Check sheet for the modelled part. Datum: model origin and axes. Units: mm. Face numbers are marked on the shaded views. A direction names the side the tool comes from. Round coordinates to 2 decimals unless told otherwise and drop trailing zeros. Order: outer loops, then holes, each group sorted by start corner. A loop starts at its lowest first (then second) coordinate and runs counter-clockwise, first axis right, second up.
Q1. Set-up check for the marked faces 1 and 2: record each of +Z, -Z, +X, -X, +Y, -Y from which the full face is reachable in a straight line by a thin tool's end or side.
Q2. Scan lines: probe 1 along Y at (x, z) = (12.7, -2.6); probe 2 along Y at (x, z) = (12, -1); probe 3 along Z at (x, y) = (41, -46). Record each from-to range of solid material in increasing order.
Q3. Cross-section at B-B on x = 139.7. Record the cut outline in (y, z).
Q4. Depth check by flat-ended pin: P1, Ø8, axis at x = 88.9, y = -19.23, coming from the -Z side; P2, Ø10, axis at x = 52.5, y = -10, coming from the -Z side; P3, Ø5, axis at x = 21.5, z = -19.5, coming from the -Y side; P4, Ø3, axis at x = 12.7, y = -19.23, coming from the -Z side. Enter the tip coordinate at first touch or a pass-through.
Q5. Cross-section at D-D on x = 41.5. Record the cut outline in (y, z).
Q6. Cross-section at C-C on y = -33. Record the cut outline in (x, z), then the cut area to 3 significant figures.
Q7. Cross-section at A-A on x = 12.7. Record the cut outline in (y, z).
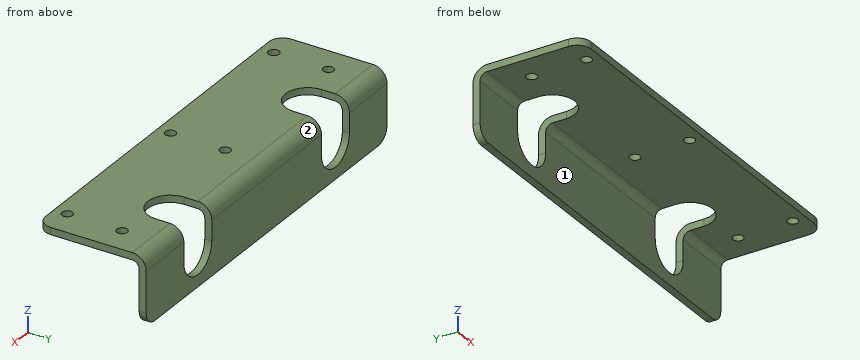
from build123d import *

# Parameters (mm, degrees)
BASE_FLANGE1_DEPTH           = 177.8
CUT_EXTRUDE1_DEPTH           = 6.5278
F_10_0_1935_DIAMETER_HOLE1_D = 4.9149
FILLET1_R                    = 6.35
CUT_EXTRUDE2_DEPTH           = 3.2639


# Sheet-metal steps are written as plain solids
with BuildPart() as part:
    # Sketch1 → Base-Flange1 (new body)
    with BuildSketch(Plane(origin=(0, 0, 0), x_dir=(0, 0, -1), z_dir=(1, 0, 0))):
        with BuildLine():
            Line((31.75, 0), (6.5278, 0))
            ThreePointArc((6.5278, 0), (1.911948354, -1.911948354), (0, -6.5278))
            Line((0, -6.5278), (0, -50.8))
            Line((0, -50.8), (3.2639, -50.8))
            Line((3.2639, -50.8), (3.2639, -6.5278))
            ThreePointArc((3.2639, -6.5278), (4.219874177, -4.219874177), (6.5278, -3.2639))
            Line((6.5278, -3.2639), (31.75, -3.2639))
            Line((31.75, -3.2639), (31.75, 0))
        make_face()
    extrude(amount=BASE_FLANGE1_DEPTH)

    # Sketch6 → Cut-Extrude1 (cut)
    with BuildSketch(Plane(origin=(0, 0, 0), x_dir=(1, 0, 0), z_dir=(0, 1, 0))):
        with BuildLine():
            Line((27.78125, 0), (27.78125, 15.875))
            ThreePointArc((27.78125, 15.875), (38.1, 26.19375), (48.41875, 15.875))
            Line((48.41875, 15.875), (48.41875, 0))
            ThreePointArc((48.41875, 0), (38.1, -10.31875), (27.78125, 0))
        make_face()
        with BuildLine():
            Line((129.38125, 0), (129.38125, 15.875))
            ThreePointArc((129.38125, 15.875), (139.7, 26.19375), (150.01875, 15.875))
            Line((150.01875, 15.875), (150.01875, 0))
            ThreePointArc((150.01875, 0), (139.7, -10.31875), (129.38125, 0))
        make_face()
    extrude(amount=-CUT_EXTRUDE1_DEPTH, mode=Mode.SUBTRACT)

    # #10 (0.1935) Diameter Hole1 (through all)
    with Locations(Plane.XY):
        with Locations((12.7, -19.2278), (88.9, -19.2278), (165.1, -19.2278), (88.9, -44.6278), (165.1, -44.6278), (12.7, -44.6278)):
            Hole(F_10_0_1935_DIAMETER_HOLE1_D / 2)

    # Fillet1
    fillet1_edges = [part.edges().sort_by_distance(p)[0] for p in [
        (177.8, -50.8, -1.63195),
        (0, -50.8, -1.63195),
        (177.8, -1.63195, -31.75),
        (0, -1.63195, -31.75),
    ]]
    fillet(fillet1_edges, radius=FILLET1_R)

    # Sketch9 → Cut-Extrude2 (cut)
    with BuildSketch(Plane.XY):
        with BuildLine():
            Line((48.41875, -6.5278), (48.41875, -12.8778))
            ThreePointArc((48.41875, -12.8778), (38.1, -23.19655), (27.78125, -12.8778))
            Line((27.78125, -12.8778), (27.78125, -6.5278))
            ThreePointArc((27.78125, -6.5278), (38.1, 3.79095), (48.41875, -6.5278))
        make_face()
        with BuildLine():
            Line((150.01875, -6.5278), (150.01875, -12.8778))
            ThreePointArc((150.01875, -12.8778), (139.7, -23.19655), (129.38125, -12.8778))
            Line((129.38125, -12.8778), (129.38125, -6.5278))
            ThreePointArc((129.38125, -6.5278), (139.7, 3.79095), (150.01875, -6.5278))
        make_face()
    extrude(amount=-CUT_EXTRUDE2_DEPTH, mode=Mode.SUBTRACT)


solid = part.part
Results found:
1. face 1: -Z, +X, -X, -Y
1. face 2: +Z, +X, -X, +Y
2. probe 1: y = -50.8 to -47.09, -42.17 to -21.69, -16.77 to -1.31
2. probe 2: y = -50.8 to -46.98, -42.27 to -21.58, -16.87 to -3.06
2. probe 3: z = -3.26 to 0
3. outline: (-50.8, -3.26) - (-23.2, -3.26) - (-23.2, 0) - (-50.8, 0) - close; (-3.26, -31.75) - (0, -31.75) - (0, -26.19) - (-3.26, -26.19) - close
4. P1: stops at z = -3.26
4. P2: stops at z = -3.64
4. P3: stops at y = -3.26
4. P4: passes through
5. outline: (-50.8, -3.26) - (-22.62, -3.26) - (-22.62, 0) - (-50.8, 0) - close; (-3.26, -31.75) - (0, -31.75) - (0, -25.62) - (-3.26, -25.62) - close
6. outline: (0, -3.26) - (177.8, -3.26) - (177.8, 0) - (0, 0) - close
6. area: 580 mm2
7. outline: (-50.8, -3.26) - (-47.09, -3.26) - (-47.09, 0) - (-50.8, 0) - close; (-42.17, -3.26) - (-21.69, -3.26) - (-21.69, 0) - (-42.17, 0) - close; (-16.77, -3.26) - (-6.53, -3.26) arc R3.26 cw to (-3.26, -6.53) - (-3.26, -31.75) - (0, -31.75) - (0, -6.53) arc R6.53 ccw to (-6.53, 0) - (-16.77, 0) - close
